Can you work these out from the model? Positions are in its coordinate system, mm. A direction names the side the tool comes from. Round coordinates to 2 decimals unless told otherwise and drop trailing zeros. Write each loop counter-clockwise with the first axis right and the second up, starting at its lowest first coordinate (ties: lowest second). Pieces come first, ordered by that corner, then holes.
Q1. Please list where these lines run through material, in increasing order: line 1 along Y through (x, z) = (23, -12); line 2 along X through (y, z) = (25, 16.5); line 3 along Z through (x, y) = (17, 17.5).
Q2. If we section it at D-D (y = 12.5): Please give me the cut outline in (x, z), plus the area to 3 significant figures.
Q3. I'm going to push flat-ended pins straight in: pin 1 Ø15.5 at (x, y) = (38, 9) entering from -Z; pin 2 Ø2 at (y, z) = (29, -12.5) entering from +X; pin 3 Ø2 at (x, z) = (39, -16) entering from +Y. Where does each tip first touch, or does it pass through?
Q4. If we section it at B-B (x = -44): Please give me the cut outline in (y, z).
Q5. We'd pull the mould along Z, two halves only. Please class faces 1 (the flat face through (-49, 16, 19.023)), 2 (the cylindrical face through (13.972, 9.787, -0.218)), 3 (the flat face through (-52.324, 19, 0)), 4 (the flat face through (38, 10, 9.906)): +Z half, -Z half, draft (parallel to the pull), parting line (faces both ways), or undercut.
Q6. If we section it at A-A (y = 22): Please give me the cut outline in (x, z).
Q7. If we section it at C-C (z = 0): Please give me the cut outline in (x, y).
Q8. For faces 5 (the flat face through (-45.72, 16, -24)), 6 (the flat face through (-28.448, 26, 0)), 7 (the flat face through (-45.72, 16, 24)), 8 (the flat face through (38, 10, -9.906)), which set-ups out of +Z, -Z, +X, -X, +Y, -Y let a thin tool reach every point of the face, with its end or its side?
Autodesk Inventor part; units mm, degrees
ref_plane "YZ Plane" through (0, 0, 0) normal (1, 0, 0) x (0, 1, 0)
ref_plane "XZ Plane" through (0, 0, 0) normal (0, 1, 0) x (-1, 0, 0)
ref_plane "XY Plane" through (0, 0, 0) normal (0, 0, 1) x (1, 0, 0)
sketch "Sketch1" plane through (0, 0, 0) normal (0, 1, 0) x (-1, 0, 0)
  line L0 (-52.324, -29.21) -> (52.324, -29.21)
  line L1 (52.324, -29.21) -> (52.324, 29.21)
  line L2 (52.324, 29.21) -> (-52.324, 29.21)
  line L3 (-52.324, 29.21) -> (-52.324, -29.21)
  line L4 (-52.324, -29.21) -> (52.324, 29.21) construction
  line L5 (52.324, -29.21) -> (-52.324, 29.21) construction
  point P0 (0, 0)
  dimension "d0" = 104.648
  dimension "d1" = 58.42
extrude "Extrusion1" add sketch "Sketch1" along normal blind 38.1
sketch "Sketch2" plane through (-52.324, 0, 29.21) normal (0, 0, 1) x (1, 0, 0)
  line L0 (0, 38.1) -> (104.648, 38.1)
  line L1 (104.648, 0) -> (104.648, 38.1)
  line L2 (23.876, 38.1) -> (104.648, 38.1)
  line L3 (104.648, 38.1) -> (104.648, 19.304)
  line L4 (104.648, 19.304) -> (23.876, 19.304)
  line L5 (23.876, 19.304) -> (23.876, 38.1)
  line L6 (0, 0) -> (0, 38.1)
  line L7 (0, 0) -> (104.648, 0)
  point P0 (52.324, 0)
  dimension "d4" = 23.876
  dimension "d5" = 19.304
extrude "Extrusion2" cut sketch "Sketch2" against normal through all contours L0 L1 L4 L5
sketch "Sketch3" plane through (-52.324, 0, -29.21) normal (-1, 0, 0) x (0, 0, 1)
  line L0 (0, 38.1) -> (58.42, 38.1)
  line L1 (39.0626, 38.1) -> (58.42, 26.924)
  line L2 (58.42, 0) -> (58.42, 38.1)
  point P0 (29.21, 0)
  dimension "d8" = 11.176
  dimension "d9" = 30
extrude "Extrusion3" cut sketch "Sketch3" against normal through all
sketch "Sketch4" plane through (-52.324, 0, -29.21) normal (-1, 0, 0) x (0, 0, 1)
  line L0 (0, 38.1) -> (39.0626, 38.1)
  line L1 (19.3574, 38.1) -> (0, 26.924)
  line L2 (0, 38.1) -> (0, 19.304)
  point P0 (29.21, 0)
  dimension "d12" = 11.176
  dimension "d13" = 30
extrude "Extrusion4" cut sketch "Sketch4" against normal through all
sketch "Sketch5" plane through (-28.448, 19.304, 29.21) normal (0, 1, 0) x (1, 0, 0)
  line L0 (80.772, 0) -> (0, 0)
  line L1 (32.512, 0) -> (80.772, 11.684)
  line L2 (80.772, 58.42) -> (80.772, 0)
  point P0 (28.448, 29.21)
  dimension "d16" = 48.26
  dimension "d17" = 11.684
extrude "Extrusion5" cut sketch "Sketch5" against normal through all
sketch "Sketch6" plane through (-28.448, 19.304, -29.21) normal (0, 1, 0) x (1, 0, 0)
  line L0 (80.772, 0) -> (-23.876, 0)
  line L1 (32.512, 0) -> (80.772, -11.684)
  line L2 (80.772, 0) -> (80.772, -46.736)
  point P0 (28.448, -29.21)
  dimension "d20" = 11.684
  dimension "d21" = 48.26
extrude "Extrusion6" cut sketch "Sketch6" against normal through all
sketch "Sketch7" plane through (0, 0, 0) normal (0, -1, 0) x (1, 0, 0)
  line L0 (-52.324, 29.21) -> (-52.324, 9.8526)
  line L1 (-52.324, 19.5313) -> (-45.72, 19.5313)
  line L2 (-45.72, 19.5313) -> (-45.72, 29.6913)
  line L3 (-45.72, 29.6913) -> (-52.324, 29.6913)
  line L4 (-52.324, 29.6913) -> (-52.324, 19.5313)
  point P0 (0, 0)
  dimension "d25" = 6.604
  dimension "d26" = 10.16
extrude "Extrusion7" cut sketch "Sketch7" against normal through all
sketch "Sketch8" plane through (0, 0, 0) normal (0, -1, 0) x (1, 0, 0)
  line L0 (-52.324, -9.8526) -> (-52.324, -29.21)
  line L1 (-52.324, -19.5313) -> (-45.72, -19.5313)
  line L2 (-45.72, -19.5313) -> (-45.72, -29.6913)
  line L3 (-45.72, -29.6913) -> (-52.324, -29.6913)
  line L4 (-52.324, -29.6913) -> (-52.324, -19.5313)
  point P0 (0, 0)
  dimension "d29" = 6.604
  dimension "d30" = 10.16
extrude "Extrusion8" cut sketch "Sketch8" against normal through all
sketch "Sketch9" plane through (-28.448, 19.304, 29.21) normal (0, 1, 0) x (1, 0, 0)
  line L0 (80.772, 46.736) -> (80.772, 11.684)
  circle A0 centre (52.324, 29.21) radius 9.906
  point P0 (28.448, 29.21)
  point P1 (80.772, 29.21)
  point P2 (80.772, 29.21)
  dimension "d35" = 19.812
  dimension "d36" = 28.448
extrude "Extrusion9" cut sketch "Sketch9" against normal through all
sketch "Sketch10" plane through (-28.448, 19.304, 29.21) normal (0, 1, 0) x (1, 0, 0)
  circle A0 centre (52.324, 29.21) radius 9.906
  line L0 (80.772, 11.684) -> (80.772, 46.736)
  line L1 (52.324, 39.116) -> (80.772, 39.116)
  line L2 (80.772, 39.116) -> (80.772, 19.304)
  line L3 (80.772, 19.304) -> (52.324, 19.304)
  line L4 (52.324, 19.304) -> (52.324, 39.116)
  point P0 (28.448, 29.21)
  dimension "d39" = 19.812
extrude "Extrusion10" cut sketch "Sketch10" against normal through all contours A0 L1 L0 L3
sketch "Sketch11" plane through (0, 0, 0) normal (0, -1, 0) x (1, 0, 0)
  line L0 (-52.324, -19.5313) -> (-52.324, 19.5313)
  line L1 (-52.324, -19.5313) -> (-45.72, -19.5313)
  line L2 (-45.72, -19.5313) -> (-45.72, -19.0233)
  line L3 (-45.72, -19.0233) -> (-52.324, -19.0233)
  line L4 (-52.324, -19.0233) -> (-52.324, -19.5313)
  point P0 (0, 0)
  dimension "d42" = 0.508
sketch "Sketch12" plane through (0, 0, 0) normal (0, -1, 0) x (1, 0, 0)
  line L0 (-52.324, -19.5313) -> (-52.324, 19.5313)
  line L1 (-52.324, 19.5313) -> (-45.72, 19.5313)
  line L2 (-45.72, 19.5313) -> (-45.72, 19.0233)
  line L3 (-45.72, 19.0233) -> (-52.324, 19.0233)
  line L4 (-52.324, 19.0233) -> (-52.324, 19.5313)
  point P0 (0, 0)
  dimension "d43" = 0.508
extrude "Extrusion11" cut sketch "Sketch11" against normal through all
extrude "Extrusion12" cut sketch "Sketch12" against normal through all
properties part number "FINGER GUIDE"
A:
1. line 1: y = 0 to 19.3
1. line 2: x = -52.32 to -28.45
1. line 3: z = -26.08 to -7.13, 7.13 to 26.08
2. outline: (-52.32, -19.02) - (-45.72, -19.02) - (-45.72, -29.21) - (4.06, -29.21) - (52.32, -17.53) - (52.32, -9.91) - (23.88, -9.91) arc R9.91 cw to (23.88, 9.91) - (52.32, 9.91) - (52.32, 17.53) - (4.06, 29.21) - (-45.72, 29.21) - (-45.72, 19.02) - (-52.32, 19.02) - close
2. area: 4,700 mm2
3. pin 1: stops at z = -22.87
3. pin 2: stops at x = -28.45
3. pin 3: stops at y = 19.3
4. outline: (0, -29.21) - (26.92, -29.21) - (38.1, -9.85) - (38.1, 9.85) - (26.92, 29.21) - (0, 29.21) - close
5. face 1: +Z half
5. face 2: undercut
5. face 3: draft
5. face 4: undercut
6. outline: (-52.32, -19.02) - (-45.72, -19.02) - (-45.72, -29.21) - (-28.45, -29.21) - (-28.45, 29.21) - (-45.72, 29.21) - (-45.72, 19.02) - (-52.32, 19.02) - close
7. outline: (-52.32, 0) - (13.97, 0) - (13.97, 19.3) - (-28.45, 19.3) - (-28.45, 38.1) - (-52.32, 38.1) - close
8. face 5: -Z, -X, +Y, -Y
8. face 6: +Z, -Z, +X, +Y
8. face 7: +Z, -X, +Y, -Y
8. face 8: +X, +Y, -Y
